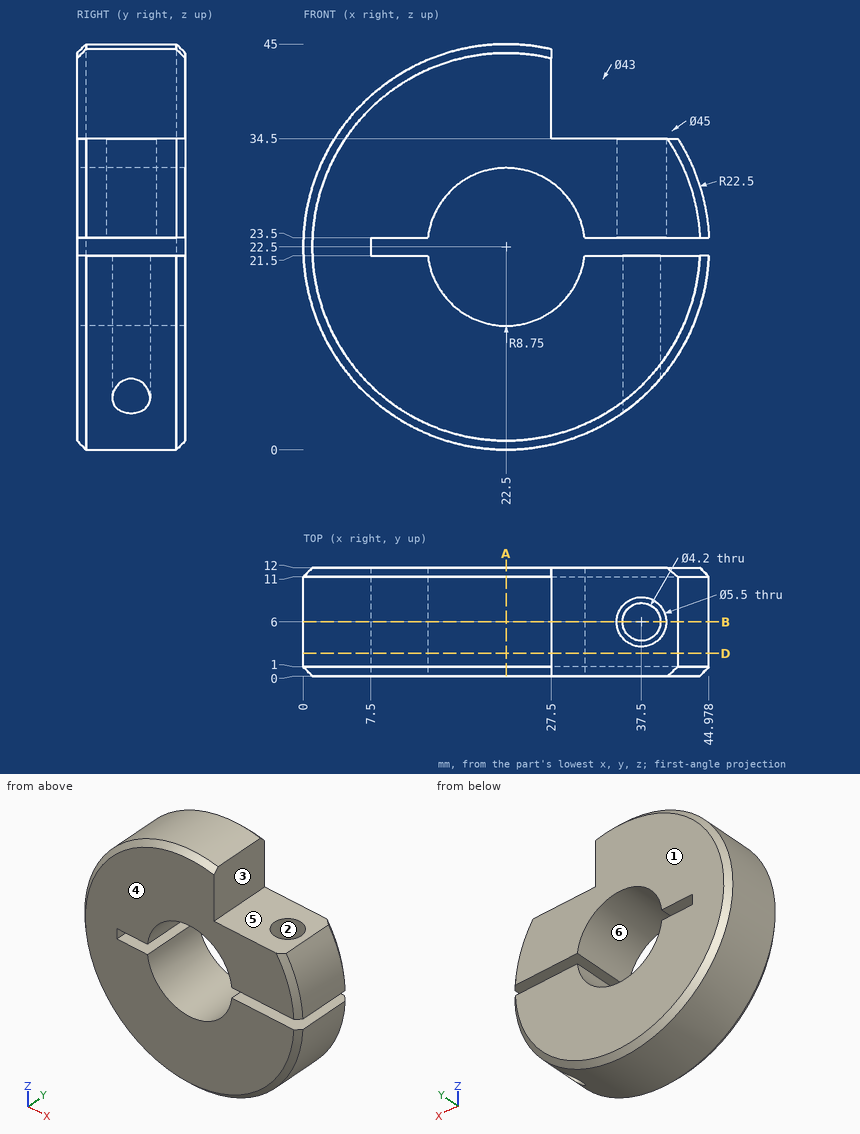
Source: three-view drawing plus pictorial views. Frame: mm from the lowest corner of the part. A direction names the side the tool comes from. Coordinates: 2 decimals unless noted, no trailing zeros. Order: outer loops, then holes, each group sorted by start corner. A loop starts at its lowest first (then second) coordinate and runs counter-clockwise, first axis right, second up.
Item 1: Cut plane D-D (y = 2.5). Return loops of the section in (x, z), plus the area to 3 significant figures.
Output values:
outline: (7.5, 21.5) - (7.5, 23.5) - (13.81, 23.5) arc R8.75 cw to (31.19, 23.5) - (44.98, 23.5) arc R22.5 ccw to (41.53, 34.5) - (27.5, 34.5) - (27.5, 44.44) arc R22.5 ccw (long way) to (44.98, 21.5) - (31.19, 21.5) arc R8.75 cw to (13.81, 21.5) - close
area: 1,220 mm2
Item 2: Material intervals for line 1 (X direction, y = 1.75, z = 25) (1 decimal); line 2 (X direction, y = 6, z = 15.75) (1 decimal); line 3 (X direction, y = 9.5, z = 26), sorted ascending.
Output values:
line 1: x = 0.1 to 14.1, 30.9 to 44.9
line 2: x = 1 to 16.9, 28.1 to 35.4, 39.6 to 44
line 3: x = 0.27 to 14.48, 30.52 to 44.73
Item 3: Cut plane B-B (y = 6). Count the separate pieces of the cut face and the enclosed holes in it, plus the area to 3 significant figures.
Output values:
separate pieces: 3
enclosed holes: 0
area: 1,090 mm2
Item 4: Pull-direction query (Y, two-part tool) for the marked faces 1, 2 and 3; classes: pulls with the +Y half, pulls with the -Y half, needs draft (parallel to the pull), parting line crosses it, or undercut.
Output values:
face 1: pulls with the +Y half
face 2: undercut
face 3: needs draft
Item 5: Set-up query: the marked faces 4, 5 and 6. Return all of +Z, -Z, +X, -X, +Y, -Y with unobstructed straight access to the full face (end or side cutting, diameter ignored); none if empty.
Output values:
face 4: +Z, -Z, +X, -X, -Y
face 5: +Z, +X, +Y, -Y
face 6: +Y, -Y
Item 6: First-contact query: P1, Ø5, axis at y = 4.5, z = 41, coming from the +X side; P2, Ø2, axis at y = 8, z = 27, coming from the -X side; P3, Ø1, axis at y = 3, z = 37, coming from the -X side; P4, Ø8, axis at x = 36, z = 34, coming from the -Y side. Flat tips, straight axial feed; report the tip coordinate or a pass-through.
Output values:
P1: stops at x = 27.5
P2: stops at x = 0.27
P3: stops at x = 4.89
P4: stops at y = 0
Item 7: Cut plane A-A (x = 22.5). Return loops of the section in (y, z), plus the area to 3 significant figures.
Output values:
outline: (0, 1) - (1, 0) - (11, 0) - (12, 1) - (12, 13.75) - (0, 13.75) - close; (0, 31.25) - (12, 31.25) - (12, 44) - (11, 45) - (1, 45) - (0, 44) - close
area: 328 mm2
